The listing builds one solid part. Answer for the finished solid, in the listing's coordinates (mm). A direction names the side the tool comes from. Coordinates: 2 decimals unless noted, no trailing zeros. Order: outer loops, then holes, each group sorted by start corner. A loop starts at its lowest first (then second) coordinate and runs counter-clockwise, first axis right, second up. Notation, with made-up numbers: (30, -4) -> (74, -4) arc R30 ccw to (74, 28) -> close; hole circle Ø3 at (51.5, -12.5). An arc over 180 degrees is marked (long way). Return JSON: item names as keys, results as strings.
```python
from build123d import *

# Parameters (mm, degrees)
F0_R     = 25.4
F1_DEPTH = 50.8
F2_DEPTH = 44.45
F3_R     = 12.7
F4_DEPTH = 50.8


with BuildPart() as f1:
    # F0 (on Front) → F1 (new body)
    with BuildSketch(Plane.XZ):
        Polygon((-324.775483, -205.800596), (-265.085489, -205.800596), (-265.085489, 155.105879), (-412.146998, 268.055191), (-428.950995, 246.176162), (-324.775483, 88.584425), align=None)
        with Locations((-295.854737, -142.300596)):
            Circle(F0_R, mode=Mode.SUBTRACT)
        with Locations((-295.854737, 110.456314)):
            Circle(F0_R, mode=Mode.SUBTRACT)
        Polygon((-265.085489, -205.800596), (-258.735483, -205.800596), (-258.735483, 158.235581), (-413.315155, 276.959153), (-432.65465, 251.778873), (-428.950995, 246.176162), (-412.146998, 268.055191), (-265.085489, 155.105879), align=None)
    extrude(amount=F1_DEPTH)

    # F0 (on Front) → F2 (cut)
    with BuildSketch(Plane.XZ):
        Polygon((-324.775483, -205.800596), (-265.085489, -205.800596), (-265.085489, 155.105879), (-412.146998, 268.055191), (-428.950995, 246.176162), (-324.775483, 88.584425), align=None)
        with Locations((-295.854737, -142.300596)):
            Circle(F0_R, mode=Mode.SUBTRACT)
        with Locations((-295.854737, 110.456314)):
            Circle(F0_R, mode=Mode.SUBTRACT)
    extrude(amount=F2_DEPTH, mode=Mode.SUBTRACT)

    # F3 (on face) → F4 (join)
    with BuildSketch(Plane(origin=(0, -44.45, 0), x_dir=(-1, 0, 0), z_dir=(0, 1, 0))):
        with Locations((404.479494, 236.68493)):
            Circle(F3_R)
    extrude(amount=F4_DEPTH)


solid = f1.part
```
Item 1: The part is cut by section A-A on z = 53. Determine the outline of the cut face in (x, y), plus the area to 3 significant figures.
Answer list:
{"outline": "(-324.78, -50.8) -> (-258.74, -50.8) -> (-258.74, 0) -> (-265.09, 0) -> (-265.09, -44.45) -> (-324.78, -44.45) -> close", "area": "702 mm2"}
Item 2: The part is cut by section B-B on y = -32.5. Determine the outline of the cut face in (x, z).
Answer list:
{"outline": "(-432.65, 251.78) -> (-428.95, 246.18) -> (-412.15, 268.06) -> (-265.09, 155.11) -> (-265.09, -205.8) -> (-258.74, -205.8) -> (-258.74, 158.24) -> (-413.32, 276.96) -> close; circle Ø25.4 at (-404.48, 236.68)"}
Item 3: Flat-ended cylindrical pins translate along their axes: pin 1 (1 mm diameter, centred on x = -318.5, z = 91.5, fed in from +Y); pin 2 (6 mm diameter, centred on y = -10.5, z = 220.5, fed in from -X); pin 3 (3 mm diameter, centred on y = -47.5, z = -39.5, fed in from -X); pin 4 (12 mm diameter, centred on x = -347.5, z = 107, fed in from -Y). Find the tip coordinate at first contact, or state that the pin passes through.
Answer list:
{"pin 1": "y = -44.45", "pin 2": "x = -354.14", "pin 3": "x = -324.78", "pin 4": "through"}
Item 4: The part is cut by section C-C on x = -366.5. Determine the outline of the cut face in (y, z), plus the area to 3 significant figures.
Answer list:
{"outline": "(-50.8, 151.7) -> (-44.45, 151.7) -> (-44.45, 233) -> (0, 233) -> (0, 241) -> (-50.8, 241) -> close", "area": "923 mm2"}
Item 5: Determine the mould class of faces 1 (the flat face through (-422.85, -25.044, 264.545)), 2 (the cylindrical face through (-299.161, -47.581, -117.117)), 3 (the flat face through (-277, -46, -205.801)) for opening direction Z: pulls with the +Z half, pulls with the -Z half, needs draft (parallel to the pull), parting line crosses it, or undercut.
Answer list:
{"face 1": "pulls with the +Z half", "face 2": "undercut", "face 3": "pulls with the -Z half"}
Item 6: Which of the six approach directions +Z, -Z, +X, -X, +Y, -Y give full straight-line access (tool end or side, diameter ignored) to faces 4 (the cylindrical face through (-394.4, -19.41, 228.96)), 5 (the flat face through (-334.943, -25.044, 216.766)), 6 (the flat face through (-265.085, -22, -28))?
Answer list:
{"face 4": "+Y", "face 5": "+Z, +X, +Y, -Y", "face 6": "-Z, -X, +Y"}
Item 7: Find the intervals of material crossed by probe 1 along X at (y, z) = (-1, 34); probe 2 along Y at (x, z) = (-411.5, 256); probe 3 along X at (y, z) = (-9.5, 246.5), in increasing order.
Answer list:
{"probe 1": "-265.09 to -258.74", "probe 2": "-50.8 to -44.45", "probe 3": "-429.17 to -428.7, -412.54 to -396.42, -384.08 to -373.66"}
